The figure shows three views and two pictorial views of one solid part (mm, origin at its lowest corner). Answer the questions. A direction names the side the tool comes from. Give positions to 0.01 mm unless a question says otherwise; leave off trailing zeros. Write each loop counter-clockwise with the first axis right and the second up, starting at its lowest first coordinate (ties: lowest second). Pieces come first, ordered by that corner, then holes. Notation, with made-up numbers: (-6, 4.5) - (18, 4.5) arc R9 cw to (18, 14.5) - close; hole circle Ø4 at (6.25, 66.25). An arc over 180 degrees is marked (long way). Use a Markdown table: item, result. Add a question column.
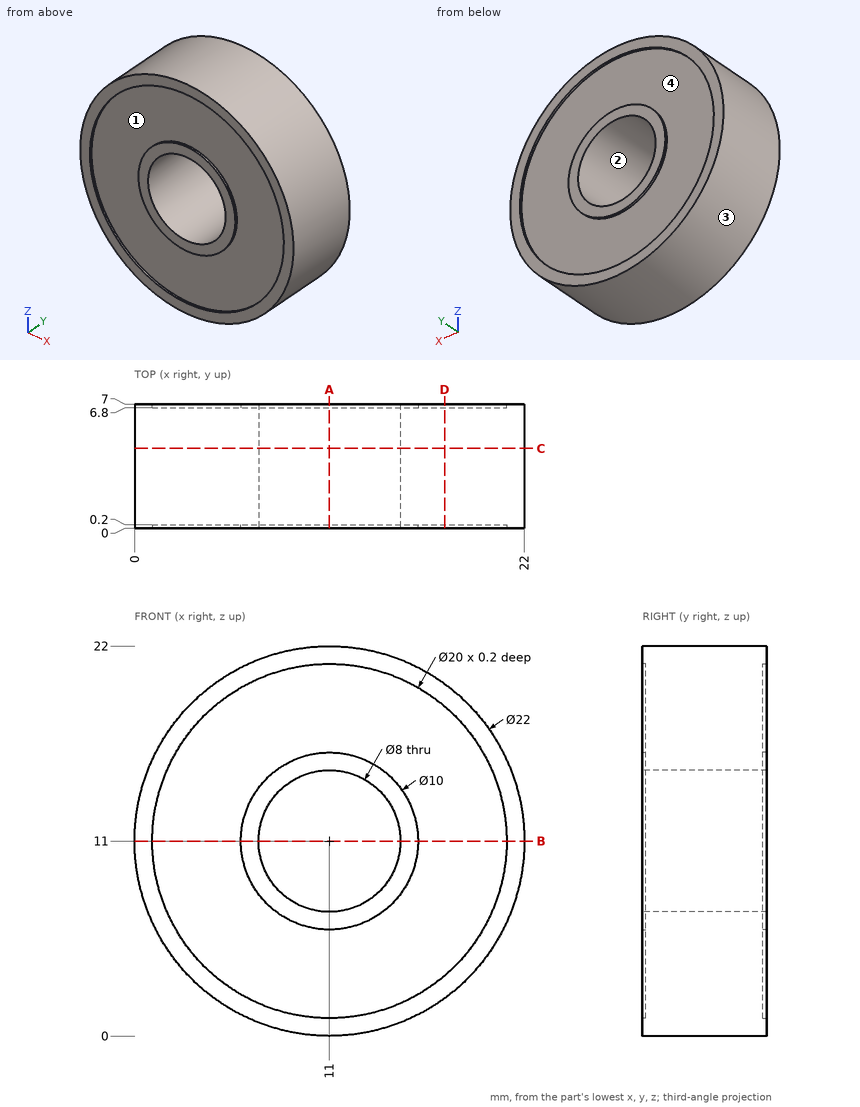
1. For a pull along Z with two mould halves and no side action, classify the marked faces 3 and 4 as released by +Z, released by -Z, zero draft, split by the parting line, or undercut.
2. The part is cut by section D-D (x = 17.5). Give the vertices of the cut face in (y, z).
3. Consider L1, parallel to X at y = 0.15, z = 11; L2, parallel to Z at x = 11, y = 3.75. Determine where each line is inside the solid, lowest interval first. Write a range as [from, to].
4. Given P1, Ø2, axis at y = 4.5, z = 7.5, coming from the -X side; P2, Ø2, axis at x = 7.5, z = 16.5, coming from the +Y side, each flat-ended and moving along its own axis, determine where each tip first touches the part or whether it passes through.
5. The part is cut by section C-C (y = 4.5). Give the vertices of the cut face in (x, z).
6. The part is cut by section B-B (z = 11). Give the vertices of the cut face in (x, y), and give its area (3 significant figures).
7. Which of the six approach directions +Z, -Z, +X, -X, +Y, -Y give full straight-line access (tool end or side, diameter ignored) to the marked faces 1 and 2?
8. The part is cut by section A-A (x = 11). Give the vertices of the cut face in (y, z).
Check values:
| question | item | result |
|---|---|---|
| 1 | face 3 | split by the parting line |
| 1 | face 4 | undercut |
| 2 | outline | (0, 2.13) - (7, 2.13) - (7, 3.4) - (6.8, 3.4) - (6.8, 18.6) - (7, 18.6) - (7, 19.87) - (0, 19.87) - (0, 18.6) - (0.2, 18.6) - (0.2, 3.4) - (0, 3.4) - close |
| 3 | L1 | x = [0, 1], [6, 7], [15, 16], [21, 22] |
| 3 | L2 | z = [0, 7], [15, 22] |
| 4 | P1 | stops at x = 0.29 |
| 4 | P2 | stops at y = 6.8 |
| 5 | outline | circle Ø22 at (11, 11); hole circle Ø8 at (11, 11) |
| 6 | outline | (0, 0) - (1, 0) - (1, 0.2) - (6, 0.2) - (6, 0) - (7, 0) - (7, 7) - (6, 7) - (6, 6.8) - (1, 6.8) - (1, 7) - (0, 7) - close; (15, 0) - (16, 0) - (16, 0.2) - (21, 0.2) - (21, 0) - (22, 0) - (22, 7) - (21, 7) - (21, 6.8) - (16, 6.8) - (16, 7) - (15, 7) - close |
| 6 | area | 94.0 mm2 |
| 7 | face 1 | -Y |
| 7 | face 2 | +Y, -Y |
| 8 | outline | (0, 0) - (7, 0) - (7, 1) - (6.8, 1) - (6.8, 6) - (7, 6) - (7, 7) - (0, 7) - (0, 6) - (0.2, 6) - (0.2, 1) - (0, 1) - close; (0, 15) - (7, 15) - (7, 16) - (6.8, 16) - (6.8, 21) - (7, 21) - (7, 22) - (0, 22) - (0, 21) - (0.2, 21) - (0.2, 16) - (0, 16) - close |
